Read the model definition and answer for the solid it produces. Units are mm, in the model's axes. Coordinates: 2 decimals unless noted, no trailing zeros. Write each loop counter-clockwise with the first axis right and the second up, starting at its lowest first coordinate (ties: lowest second). Pieces come first, ordered by that corner, then holes.
1) Each of these flat-tipped pins is pushed along its axis until it touches: pin 1 Ø6.5 at (x, y) = (29.5, 44.5) entering from +Z; pin 2 Ø3 at (x, y) = (29, 7) entering from +Z. Where does it stop, or does it pass through?
2) Find the intervals of material crossed by line 1 (Y direction, x = 29, z = 0.75); line 2 (X direction, y = 7, z = 0.6); line 3 (X direction, y = 43, z = 6.55), in increasing order.
3) The part is cut by section A-A (y = 43). Determine the outline of the cut face in (x, z), then the cut area to 3 significant figures.
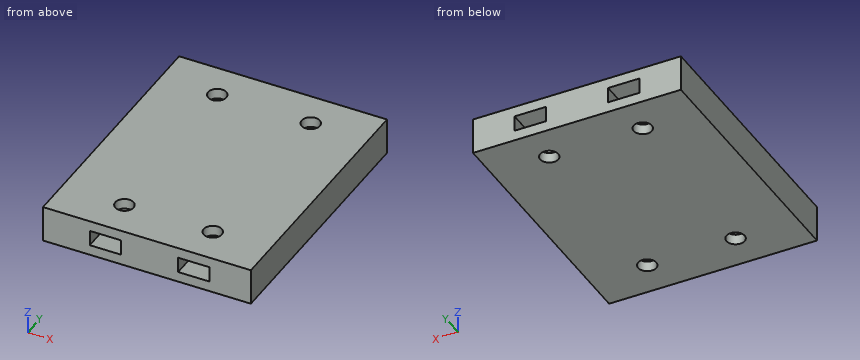
from build123d import *

# Parameters (mm, degrees)
CYLINDER021_R             = 1.75
CYLINDER021_DEPTH         = 30
BOX023_W                  = 20
BOX023_H                  = 6
BOX023_DEPTH              = 3
PRISM021_DEPTH            = 3
FUSION018_PLACEMENT_ANGLE = 90
CYLINDER019_R             = 1.75
CYLINDER019_DEPTH         = 30
BOX020_W                  = 20
BOX020_H                  = 6
BOX020_DEPTH              = 3
PRISM019_DEPTH            = 3
FUSION019_PLACEMENT_ANGLE = 90
CYLINDER022_R             = 1.75
CYLINDER022_DEPTH         = 30
BOX021_W                  = 20
BOX021_H                  = 6
BOX021_DEPTH              = 3
PRISM022_DEPTH            = 3
FUSION020_PLACEMENT_ANGLE = 90
CYLINDER020_R             = 1.75
CYLINDER020_DEPTH         = 30
BOX022_W                  = 20
BOX022_H                  = 6
BOX022_DEPTH              = 3
PRISM020_DEPTH            = 3
FUSION017_PLACEMENT_ANGLE = 90
BOX019_W                  = 40
BOX019_H                  = 50
BOX019_DEPTH              = 7


with BuildPart() as cilindro021:
    # Cylinder021 → Cylinder021 (new body)
    with BuildSketch(Plane.XY.offset(-5)):
        Circle(CYLINDER021_R)
    extrude(amount=CYLINDER021_DEPTH)


with BuildPart() as cubo023:
    # Box023 → Box023 (new body)
    with BuildSketch(Plane(origin=(1, -3, 0), x_dir=(1, 0, 0), z_dir=(0, 0, 1))):
        with Locations((10, 3)):
            Rectangle(BOX023_W, BOX023_H)
    extrude(amount=BOX023_DEPTH)


with BuildPart() as fusion018:
    # Prism021 → Prism021 (new body)
    with BuildSketch(Plane.XY):
        Polygon((3.25, 0), (1.625, 2.814583), (-1.625, 2.814583), (-3.25, 0), (-1.625, -2.814583), (1.625, -2.814583), align=None)
    extrude(amount=PRISM021_DEPTH)

    # Fusion018: union Cilindro021, Cubo023
    add(cilindro021.part)
    add(cubo023.part)


with BuildPart() as fusion018_1:
    # Fusion018 placement: moved
    add(fusion018.part.moved(Location((29, 43, 2))).rotate(Axis((29, 43, 2), (0, 0, 1)), FUSION018_PLACEMENT_ANGLE))


with BuildPart() as cilindro019:
    # Cylinder019 → Cylinder019 (new body)
    with BuildSketch(Plane.XY.offset(-5)):
        Circle(CYLINDER019_R)
    extrude(amount=CYLINDER019_DEPTH)


with BuildPart() as cubo020:
    # Box020 → Box020 (new body)
    with BuildSketch(Plane(origin=(1, -3, 0), x_dir=(1, 0, 0), z_dir=(0, 0, 1))):
        with Locations((10, 3)):
            Rectangle(BOX020_W, BOX020_H)
    extrude(amount=BOX020_DEPTH)


with BuildPart() as fusion019:
    # Prism019 → Prism019 (new body)
    with BuildSketch(Plane.XY):
        Polygon((3.25, 0), (1.625, 2.814583), (-1.625, 2.814583), (-3.25, 0), (-1.625, -2.814583), (1.625, -2.814583), align=None)
    extrude(amount=PRISM019_DEPTH)

    # Fusion019: union Cilindro019, Cubo020
    add(cilindro019.part)
    add(cubo020.part)


with BuildPart() as fusion019_1:
    # Fusion019 placement: moved
    add(fusion019.part.moved(Location((29, 7, 2))).rotate(Axis((29, 7, 2), (0, 0, -1)), FUSION019_PLACEMENT_ANGLE))


with BuildPart() as cilindro022:
    # Cylinder022 → Cylinder022 (new body)
    with BuildSketch(Plane.XY.offset(-5)):
        Circle(CYLINDER022_R)
    extrude(amount=CYLINDER022_DEPTH)


with BuildPart() as cubo021:
    # Box021 → Box021 (new body)
    with BuildSketch(Plane(origin=(1, -3, 0), x_dir=(1, 0, 0), z_dir=(0, 0, 1))):
        with Locations((10, 3)):
            Rectangle(BOX021_W, BOX021_H)
    extrude(amount=BOX021_DEPTH)


with BuildPart() as fusion020:
    # Prism022 → Prism022 (new body)
    with BuildSketch(Plane.XY):
        Polygon((3.25, 0), (1.625, 2.814583), (-1.625, 2.814583), (-3.25, 0), (-1.625, -2.814583), (1.625, -2.814583), align=None)
    extrude(amount=PRISM022_DEPTH)

    # Fusion020: union Cilindro022, Cubo021
    add(cilindro022.part)
    add(cubo021.part)


with BuildPart() as fusion020_1:
    # Fusion020 placement: moved
    add(fusion020.part.moved(Location((12, 7, 2))).rotate(Axis((12, 7, 2), (0, 0, -1)), FUSION020_PLACEMENT_ANGLE))


with BuildPart() as cilindro020:
    # Cylinder020 → Cylinder020 (new body)
    with BuildSketch(Plane.XY.offset(-5)):
        Circle(CYLINDER020_R)
    extrude(amount=CYLINDER020_DEPTH)


with BuildPart() as cubo022:
    # Box022 → Box022 (new body)
    with BuildSketch(Plane(origin=(1, -3, 0), x_dir=(1, 0, 0), z_dir=(0, 0, 1))):
        with Locations((10, 3)):
            Rectangle(BOX022_W, BOX022_H)
    extrude(amount=BOX022_DEPTH)


with BuildPart() as fusion017:
    # Prism020 → Prism020 (new body)
    with BuildSketch(Plane.XY):
        Polygon((3.25, 0), (1.625, 2.814583), (-1.625, 2.814583), (-3.25, 0), (-1.625, -2.814583), (1.625, -2.814583), align=None)
    extrude(amount=PRISM020_DEPTH)

    # Fusion017: union Cilindro020, Cubo022
    add(cilindro020.part)
    add(cubo022.part)


with BuildPart() as fusion017_1:
    # Fusion017 placement: moved
    add(fusion017.part.moved(Location((11, 43, 2))).rotate(Axis((11, 43, 2), (0, 0, 1)), FUSION017_PLACEMENT_ANGLE))


with BuildPart() as cut029:
    # Box019 → Box019 (new body)
    with BuildSketch(Plane.XY):
        with Locations((20, 25)):
            Rectangle(BOX019_W, BOX019_H)
    extrude(amount=BOX019_DEPTH)

    # Cut026: cut Fusion017
    add(fusion017_1.part, mode=Mode.SUBTRACT)

    # Cut027: cut Fusion020
    add(fusion020_1.part, mode=Mode.SUBTRACT)

    # Cut028: cut Fusion019
    add(fusion019_1.part, mode=Mode.SUBTRACT)

    # Cut029: cut Fusion018
    add(fusion018_1.part, mode=Mode.SUBTRACT)


solid = cut029.part
Reported:
1. pin 1: stops at z = 7
1. pin 2: passes through
2. line 1: y = 0 to 5.25, 8.75 to 41.25, 44.75 to 50
2. line 2: x = 0 to 10.25, 13.75 to 27.25, 30.75 to 40
2. line 3: x = 0 to 9.25, 12.75 to 27.25, 30.75 to 40
3. outline: (0, 0) - (9.25, 0) - (9.25, 2) - (8.19, 2) - (8.19, 5) - (9.25, 5) - (9.25, 7) - (0, 7) - close; (12.75, 0) - (27.25, 0) - (27.25, 2) - (26.19, 2) - (26.19, 5) - (27.25, 5) - (27.25, 7) - (12.75, 7) - (12.75, 5) - (13.81, 5) - (13.81, 2) - (12.75, 2) - close; (30.75, 0) - (40, 0) - (40, 7) - (30.75, 7) - (30.75, 5) - (31.81, 5) - (31.81, 2) - (30.75, 2) - close
3. area: 218 mm2
